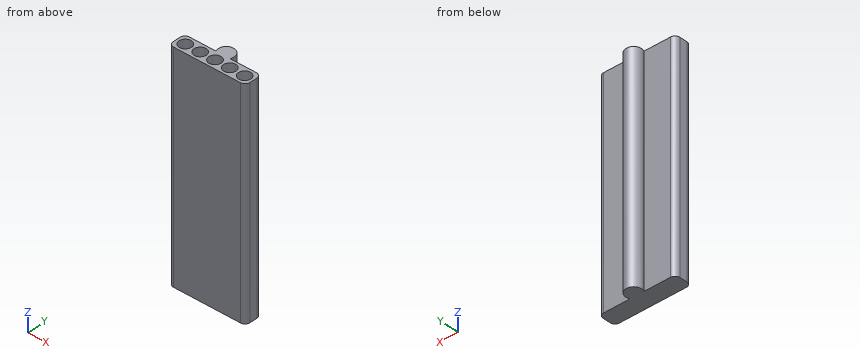
from build123d import *

# Parameters (mm, degrees)
F0_R     = 3.96875
F1_DEPTH = 139.7
F2_DEPTH = 25.4
F3_R     = 3.175


with BuildPart() as f1:
    # F0 (on Top) → F1 (new body)
    with BuildSketch(Plane.XY):
        with BuildLine():
            Line((24.60625, -44.219091), (4.524876, -44.219091))
            ThreePointArc((4.524876, -44.219091), (0, -36.83), (-4.524876, -44.219091))
            Line((-4.524876, -44.219091), (-24.60625, -44.219091))
            Line((-24.60625, -44.219091), (-24.60625, -55.331591))
            Line((-24.60625, -55.331591), (24.60625, -55.331591))
            Line((24.60625, -55.331591), (24.60625, -44.219091))
        make_face()
        with Locations((-19.05, -49.775341)):
            Circle(F0_R, mode=Mode.SUBTRACT)
        with Locations((-9.525, -49.775341)):
            Circle(F0_R, mode=Mode.SUBTRACT)
        with Locations((0, -49.775341)):
            Circle(F0_R, mode=Mode.SUBTRACT)
        with Locations((9.525, -49.775341)):
            Circle(F0_R, mode=Mode.SUBTRACT)
        with Locations((19.05, -49.775341)):
            Circle(F0_R, mode=Mode.SUBTRACT)
    extrude(amount=F1_DEPTH)

    # F0 (on Top) → F2 (join)
    with BuildSketch(Plane.XY):
        with Locations((-19.05, -49.775341)):
            Circle(F0_R)
        with Locations((-9.525, -49.775341)):
            Circle(F0_R)
        with Locations((0, -49.775341)):
            Circle(F0_R)
        with Locations((9.525, -49.775341)):
            Circle(F0_R)
        with Locations((19.05, -49.775341)):
            Circle(F0_R)
    extrude(amount=F2_DEPTH)

    # F3
    f3_edges = [f1.edges().sort_by_distance(p)[0] for p in [
        (24.60625, -55.331591, 69.85),
        (24.60625, -44.219091, 69.85),
        (-24.60625, -44.219091, 69.85),
        (-24.60625, -55.331591, 69.85),
    ]]
    fillet(f3_edges, radius=F3_R)


solid = f1.part
Input: part model. Units: mm. Frame: model coordinates. Coordinates: 2 decimals unless noted, no trailing zeros. Write each loop counter-clockwise with the first axis right and the second up, starting at its lowest first coordinate (ties: lowest second). Pieces come first, ordered by that corner, then holes. Notation, with made-up numbers: M 31,-2.5 L 42,-2.5 A14 cw 42,22.5 Z; hole C 22.25,-11 d7. An arc over 180 degrees is marked long. Answer as a JSON object with one key per item and string values. Group by question number.
(1) Ray query, line 1 along X through (y, z) = (-49.5, 44); line 2 along X through (y, z) = (-46.5, 36); line 3 along Y through (x, z) = (0, 115). Return the intervals inside material, ascending. Write a range as [from, to].
(2) Section A-A on x = 19.05. Output: boundary loops of the cut face in (y, z), plus the area to 3 significant figures.
(3) Section C-C on z = 105. Give the number of separate pieces and of enclosed holes in the cut face, plus the area to 3 significant figures.
(4) Contact query for flat-ended pins moving along their axis: P1, Ø8, axis at y = -40, z = 61, coming from the +X side; P2, Ø1, axis at x = -6.5, y = -46.5, coming from the -Z side; P3, Ø4, axis at x = 19, y = -51.5, coming from the +Z side; P4, Ø13.5, axis at x = -14.5, z = 42.5, coming from the +Y side. Output: stop coordinate, or through.
(5) Section D-D on x = 0. Output: boundary loops of the cut face in (y, z).
(6) Section B-B on y = -41.91. Output: boundary loops of the cut face in (x, z).
Result set:
{
 "1": {"line 1": "x = [-24.61, -23.01], [-15.09, -13.48], [-5.57, -3.96], [3.96, 5.57], [13.48, 15.09], [23.01, 24.61]", "line 2": "x = [-24.48, -21.29], [-16.81, -11.77], [-7.28, -2.24], [2.24, 7.28], [11.77, 16.81], [21.29, 24.48]", "line 3": "y = [-55.33, -53.74], [-45.81, -36.83]"},
 "2": {"outline": "M -55.33,0 L -44.22,0 L -44.22,139.7 L -45.81,139.7 L -45.81,25.4 L -53.74,25.4 L -53.74,139.7 L -55.33,139.7 Z", "area": "645 mm2"},
 "3": {"separate pieces": "1", "enclosed holes": "5", "area": "354 mm2"},
 "4": {"P1": "stops at x = 5.08", "P2": "stops at z = 0", "P3": "stops at z = 25.4", "P4": "stops at y = -44.22"},
 "5": {"outline": "M -55.33,0 L -36.83,0 L -36.83,139.7 L -45.81,139.7 L -45.81,25.4 L -53.74,25.4 L -53.74,139.7 L -55.33,139.7 Z"},
 "6": {"outline": "M -5.08,0 L 5.08,0 L 5.08,139.7 L -5.08,139.7 Z"}
}
